For this review, use the dimensioned drawing (mm, ordinates from the lowest corner) and the shaded views. A direction names the side the tool comes from. Give positions to 0.01 mm unless a question says otherwise; leave off trailing zeros. Loops run counter-clockwise (first coordinate to the right, second up) from the corner with the lowest first, then second, coordinate; pieces in that order, holes last. Notation, with made-up numbers: M -24.75,87 L -10.75,87 A18 ccw -10.75,101 Z; hole C -33.5,4 d10. An arc over 180 degrees is marked long. Use a Markdown table: item, result. Add a question column.
(1) Add section A-A, the plane x = 54.5. Give the boundary of the cut face in (y, z).
(2) Add section D-D, the plane z = 19.75. Give the boundary of the cut face in (x, y), then the cut area to 3 significant figures.
(3) Insertion check: pin 1 Ø10 at (x, y) = (29.5, 5) entering from +Z; pin 2 Ø3.5 at (y, z) = (4.5, 9.5) entering from +X; pin 3 Ø11 at (x, z) = (7, 6) entering from +Y; pin 4 Ø5.5 at (x, y) = (17, 8.5) entering from +Z. Each pin has a flat end and moves straight along its axis. Give the tip position at first contact, or say it passes through.
(4) For probe 1 along X at (y, z) = (13, 6); probe 2 along X at (y, z) = (2.15, 6); probe 3 along Z at (x, y) = (7, 1.85), list the stretches that pass through material, from the lowest coordinate up.
(5) For the marked faces 1, 2, 3, 4 and 5, list the 3-axis set-ups (+Z, -Z, +X, -X, +Y, -Y) from which the entire face can be reached by the end or side of a thin tool; tool diameter is ignored.
(6) Add section B-B, the plane z = 6. Give the boundary of the cut face in (x, y), then the cut area to 3 significant figures.
(7) Draft analysis for pull direction Z (two halves, no side actions). For the marked faces 6, 7, 8 and 9, state which applies: pulls with the +Z half, pulls with the -Z half, needs draft (parallel to the pull), parting line crosses it, or undercut.
(8) Add section C-C, the plane x = 39. Give the boundary of the cut face in (y, z), then the cut area to 3 significant figures.
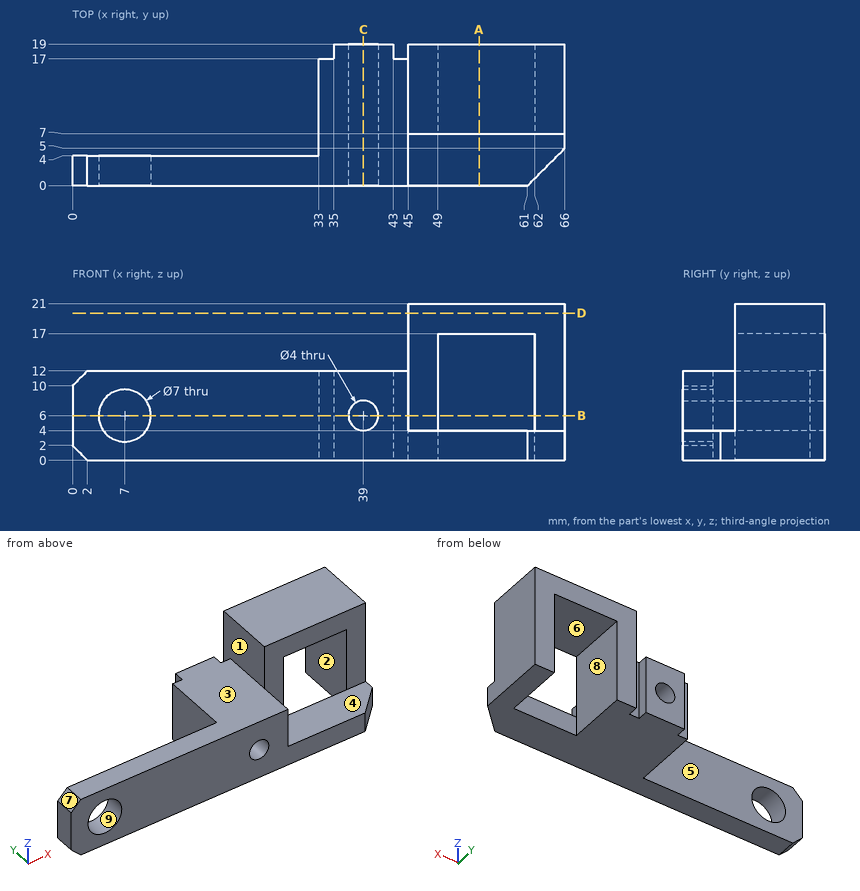
Established:
| question | item | result |
|---|---|---|
| 1 | outline | M 0,0 L 7,0 L 7,4 L 0,4 Z; M 7,17 L 19,17 L 19,21 L 7,21 Z |
| 2 | outline | M 45,7 L 66,7 L 66,19 L 45,19 Z |
| 2 | area | 252 mm^2 |
| 3 | pin 1 | z = 12 |
| 3 | pin 2 | x = 45 |
| 3 | pin 3 | y = 4 |
| 3 | pin 4 | through |
| 4 | probe 1 | 33 to 37, 41 to 49, 62 to 66 |
| 4 | probe 2 | 0 to 3.5, 10.5 to 37, 41 to 45 |
| 4 | probe 3 | 0 to 2.5, 9.5 to 12 |
| 5 | face 1 | +Z, +Y |
| 5 | face 2 | -Z, +Y |
| 5 | face 3 | +Z, -X, +Y, -Y |
| 5 | face 4 | +Z, +X, -Y |
| 5 | face 5 | +Z, -Z, -X, +Y |
| 6 | outline | M 0,0 L 3.5,0 L 3.5,4 L 0,4 Z; M 10.5,0 L 37,0 L 37,19 L 35,19 L 35,17 L 33,17 L 33,4 L 10.5,4 Z; M 41,0 L 45,0 L 45,7 L 49,7 L 49,19 L 45,19 L 45,17 L 43,17 L 43,19 L 41,19 Z; M 62,7 L 66,7 L 66,19 L 62,19 Z |
| 6 | area | 344 mm^2 |
| 7 | face 6 | pulls with the -Z half |
| 7 | face 7 | pulls with the +Z half |
| 7 | face 8 | needs draft |
| 7 | face 9 | undercut |
| 8 | outline | M 0,0 L 19,0 L 19,4 L 0,4 Z; M 0,8 L 19,8 L 19,12 L 0,12 Z |
| 8 | area | 152 mm^2 |
